Could you check a few things on this drawing? It's one solid part, dimensions in mm from its lowest x, y, z. A direction names the side the tool comes from. Give positions to 0.01 mm unless a question says otherwise; leave off trailing zeros. Loops run counter-clockwise (first coordinate to the right, second up) from the corner with the lowest first, then second, coordinate; pieces in that order, holes last.
1. Imagine slicing it at D-D (x = 3). List the corners of the cut face in (y, z) for me, plus the area to 3 significant figures.
2. Imagine slicing it at C-C (x = 13.5). List the corners of the cut face in (y, z) for me.
3. For the marked faces 1 and 2, which set-ups out of +Z, -Z, +X, -X, +Y, -Y let a thin tool reach every point of the face, with its end or its side?
4. For P1, Ø3, axis at x = 6, y = 12.5, coming from the -Z side (1 decimal); P2, Ø1, axis at x = 8.5, y = 39.5, coming from the +Z side; P3, Ø2, axis at x = 4, z = 33.5, coming from the +Y side, each with a flat end and sliding along its axis, tell me the tip position at first contact or that it passes through.
5. Imagine slicing it at A-A (y = 27). List the corners of the cut face in (x, z) for me.
6. Thinking about a two-plate mould opening in Z: for the marked faces 3, 4 and 5, which applies, +Z half, -Z half, draft (parallel to the pull), parting line (faces both ways), or undercut?
7. Imagine slicing it at B-B (z = 27). List the corners of the cut face in (x, y) for me.
8. I need wall thicknesses on line 1 along Y through (x, z) = (1.55, 27); line 2 along Y through (x, z) = (5.15, 27); line 3 along X through (y, z) = (40, 33). Which ranges of each line are inside material? Lowest first, please.
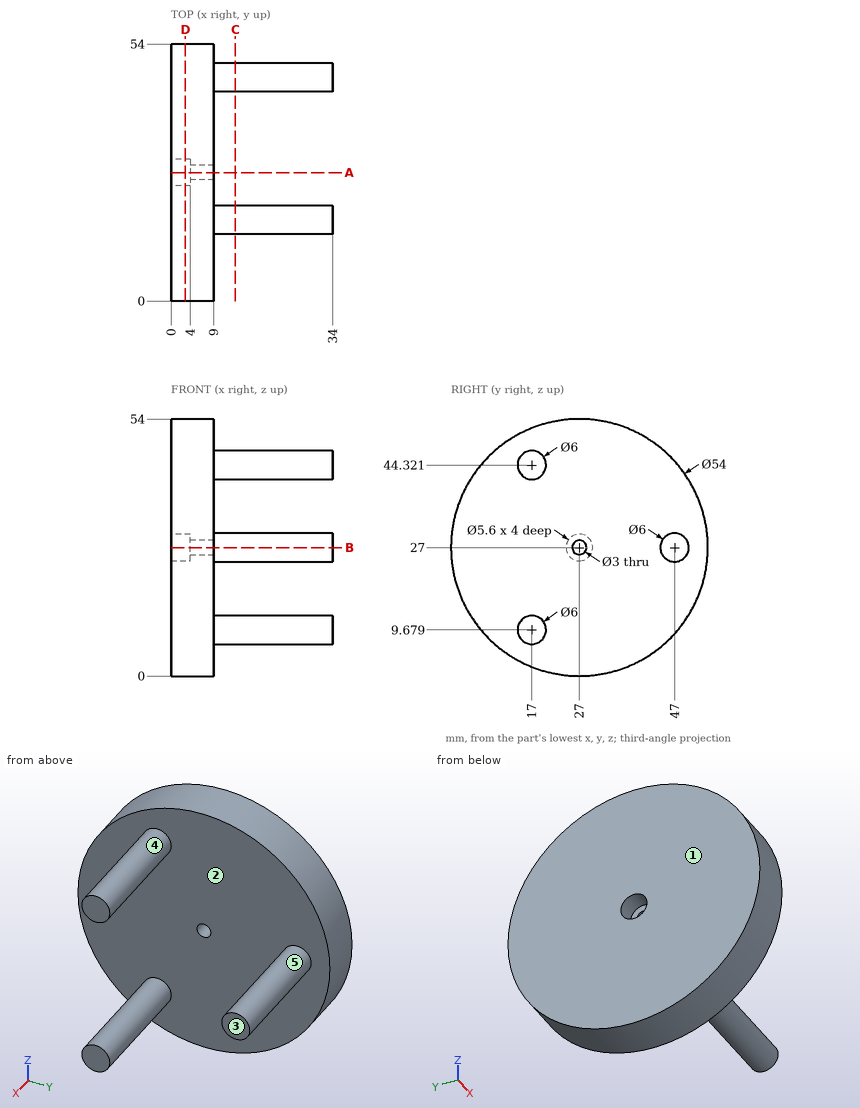
Derived:
1. outline: circle Ø54 at (27, 27); hole circle Ø5.6 at (27, 27)
1. area: 2,270 mm2
2. outline: circle Ø6 at (17, 9.68); circle Ø6 at (17, 44.32); circle Ø6 at (47, 27)
3. face 1: +Z, -Z, -X, +Y, -Y
3. face 2: +X
4. P1: stops at z = 3.3
4. P2: stops at z = 51.19
4. P3: stops at y = 53.43
5. outline: (0, 0) - (9, 0) - (9, 25.5) - (4, 25.5) - (4, 24.2) - (0, 24.2) - close; (0, 29.8) - (4, 29.8) - (4, 28.5) - (9, 28.5) - (9, 54) - (0, 54) - close
6. face 3: draft
6. face 4: undercut
6. face 5: parting line
7. outline: (0, 0) - (9, 0) - (9, 25.5) - (4, 25.5) - (4, 24.2) - (0, 24.2) - close; (0, 29.8) - (4, 29.8) - (4, 28.5) - (9, 28.5) - (9, 44) - (34, 44) - (34, 50) - (9, 50) - (9, 54) - (0, 54) - close
8. line 1: y = 0 to 24.2, 29.8 to 54
8. line 2: y = 0 to 25.5, 28.5 to 54
8. line 3: x = 0 to 9
